Design review of the part built by this model. Coordinates are the model's own, in mm. Face numbers are marked on the shaded views. A direction names the side the tool comes from. Give positions to 0.01 mm unless a question says otherwise; leave off trailing zeros. Loops run counter-clockwise (first coordinate to the right, second up) from the corner with the lowest first, then second, coordinate; pieces in that order, holes last. Notation, with made-up numbers: M 13.25,30.5 L 53.25,30.5 A18 ccw 53.25,39.5 Z; hole C 2,-28 d1. An arc over 180 degrees is marked long. Use CSV: the item, a comma, the result in double quotes.
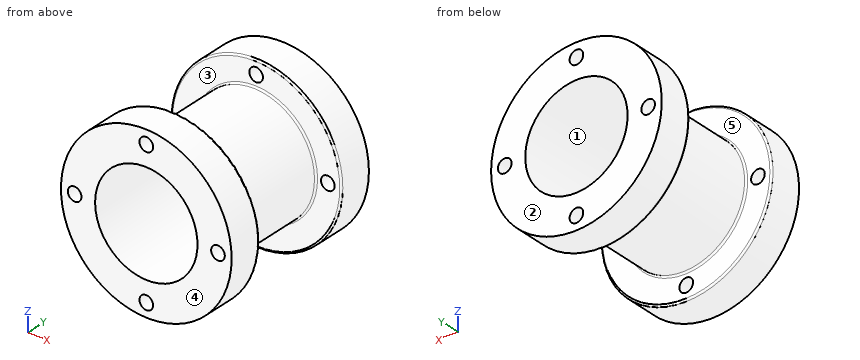
from build123d import *

# Parameters (mm, degrees)
F0_R     = 35
F1_DEPTH = 30
F3_R     = 50
F4_DEPTH = 20
F6_R     = 50
F7_DEPTH = 20
F9_D     = 60
F11_D    = 8
F12_R    = 1


with BuildPart() as f1:
    # F0 (on Front) → F1 (new body, symmetric)
    with BuildSketch(Plane.XZ):
        Circle(F0_R)
    extrude(amount=F1_DEPTH, both=True)

    # F3 (on offset) → F4 (join)
    with BuildSketch(Plane.XZ.offset(30)):
        Circle(F3_R)
    extrude(amount=F4_DEPTH)

    # F6 (on offset) → F7 (join)
    with BuildSketch(Plane.XZ.offset(-30)):
        Circle(F6_R)
    extrude(amount=-F7_DEPTH)

    # F9 (through all)
    with Locations(Plane.XZ.offset(50)):
        with Locations((0, 0)):
            Hole(F9_D / 2)

    # F11 (through all)
    with Locations(Plane.XZ.offset(50)):
        with Locations((0, 42), (-42, 0), (0, -42), (42, 0)):
            Hole(F11_D / 2)

    # F12
    f12_edges = [f1.edges().sort_by_distance(p)[0] for p in [
        (-35, -30, 0),
        (-35, 30, 0),
        (-50, 30, 0),
        (-50, -30, 0),
    ]]
    fillet(f12_edges, radius=F12_R)


solid = f1.part
(1) Clearance check with flat-ended pins moving along their axes: P1, Ø3, axis at y = 32, z = -29.5, coming from the +X side; P2, Ø5, axis at x = 42, z = 0, coming from the +Y side; P3, Ø3, axis at x = 1.5, y = -5.5, coming from the +Z side; P4, Ø3, axis at y = -34, z = 34.5, coming from the -X side. State where each tip first meets the part, or that it passes through.
A:
P1,"x = 41.42"
P2,"through"
P3,"z = 35"
P4,"x = -37.56"
(2) We need section B-B on x = 0. Count the separate pieces of the cut face and the enclosed holes in it, then the cut area to 3 significant figures.
A:
separate pieces,"6"
enclosed holes,"0"
area,"1,560 mm²"
(3) Machinability: for the marked faces 4 and 5, which of the approach directions +Z, -Z, +X, -X, +Y, -Y give a long, thin tool a straight path to every point of the face, cutting with its end or side? Answer none if there is none.
A:
face 4,"+Z, -Z, +X, -X, -Y"
face 5,"none"
(4) The part is to be moulded in two halves that separate along Y. For the marked faces 1, 2 and 3, say which applies: released by +Y, released by -Y, zero draft, split by the parting line, or undercut.
A:
face 1,"zero draft"
face 2,"released by +Y"
face 3,"undercut"
(5) We need section C-C on y = 7. State the section outline as (x, z) points, then the cut area to 3 significant figures.
A:
outline,"C 0,0 d70; hole C 0,0 d60"
area,"1,020 mm²"
(6) We need section A-A on y = 42. State the section outline as (x, z) points, then the cut area to 3 significant figures.
A:
outline,"C 0,0 d100; hole C -42,0 d8; hole C 0,0 d60; hole C 0,-42 d8; hole C 0,42 d8; hole C 42,0 d8"
area,"4,830 mm²"
(7) Wall thickness on line 1 along Z through (x, y) = (0, 40); line 2 along Z through (x, y) = (0, -16.5); line 3 along Y through (x, z) = (31.5, -18): over which ranges is each line inside the solid? List them lowest first. Write a range as [from, to].
A:
line 1,"[-50, -46], [-38, -30], [30, 38], [46, 50]"
line 2,"[-35, -30], [30, 35]"
line 3,"[-50, -30], [30, 50]"
